Here's how the part is built. I have some questions about the finished solid (model axes, mm). A direction names the side the tool comes from. Coordinates: 2 decimals unless noted, no trailing zeros. Order: outer loops, then holes, each group sorted by start corner. A loop starts at its lowest first (then second) coordinate and runs counter-clockwise, first axis right, second up.
```python
from build123d import *

# Parameters (mm, degrees)
MODEL_R                 = 8
MODEL_R_2               = 6
MODEL_W                 = 5
MODEL_H                 = 5
SALIENTE_EXTRUIR1_DEPTH = 3


with BuildPart() as part:
    # Model → Saliente-Extruir1 (new body)
    with BuildSketch(Plane.XY):
        with BuildLine():
            Line((76.347655659, 34.880000028), (76.347655659, 24.880000028))
            Line((76.347655659, 24.880000028), (73.347655659, 24.880000028))
            Line((73.347655659, 24.880000028), (73.347655659, 6.880000028))
            Line((73.347655659, 6.880000028), (76.347655659, 6.880000028))
            Line((76.347655659, 6.880000028), (76.347655659, -3.119999972))
            Line((76.347655659, -3.119999972), (73.347655659, -3.119999972))
            Line((73.347655659, -3.119999972), (73.347655659, -14.119999972))
            Line((73.347655659, -14.119999972), (61.82755788, -14.119999972))
            Line((61.82755788, -14.119999972), (5.822580598, -14.119999972))
            ThreePointArc((5.822580598, -14.119999972), (0.393738877, -12.632215144), (-3.517289733, -8.583798005))
            ThreePointArc((-3.517289733, -8.583798005), (-0.871613495, -9.225522901), (1.80545298, -8.730822292))
            ThreePointArc((1.80545298, -8.730822292), (-2.833232138, -3.402025371), (-5.249801899, 3.236774734))
            ThreePointArc((-5.249801899, 3.236774734), (-2.74505386, 2.21277877), (-0.249855047, 3.259828604))
            ThreePointArc((-0.249855047, 3.259828604), (-3.624986156, 7.837335992), (-5.559793418, 13.185382809))
            ThreePointArc((-5.559793418, 13.185382809), (-0.86111803, 15.262797511), (2.412456901, 19.222205222))
            ThreePointArc((2.412456901, 19.222205222), (-2.310766872, 27.309140745), (-4.095322699, 36.502765137))
            ThreePointArc((-4.095322699, 36.502765137), (2.717491313, 38.336145621), (6.755388207, 44.121567597))
            ThreePointArc((6.755388207, 44.121567597), (7.57877424, 45.247904396), (8.822580598, 45.880000028))
            Line((8.822580598, 45.880000028), (11.313037594, 45.880000028))
            Line((11.313037594, 45.880000028), (73.347655659, 45.880000028))
            Line((73.347655659, 45.880000028), (73.347655659, 34.880000028))
            Line((73.347655659, 34.880000028), (76.347655659, 34.880000028))
        make_face()
        with Locations((18.822580598, 28.880000028)):
            Circle(MODEL_R, mode=Mode.SUBTRACT)
        with Locations((38.822580598, 15.880000028)):
            Circle(MODEL_R_2, mode=Mode.SUBTRACT)
        with Locations((18.822580598, 2.880000028)):
            Circle(MODEL_R, mode=Mode.SUBTRACT)
        Polygon((53.725434944, 16.464936518), (56.225434944, 20.795063537), (51.895307925, 23.295063537), (49.395307925, 18.964936518), align=None, mode=Mode.SUBTRACT)
        Polygon((49.395307925, 12.795063537), (51.895307925, 8.464936518), (56.225434944, 10.964936518), (53.725434944, 15.295063537), align=None, mode=Mode.SUBTRACT)
        with Locations((59.738574665, 23.880000028)):
            Rectangle(MODEL_W, MODEL_H, mode=Mode.SUBTRACT)
        Polygon((65.751714386, 15.295063537), (63.251714386, 10.964936518), (67.581841405, 8.464936518), (70.081841405, 12.795063537), align=None, mode=Mode.SUBTRACT)
        Polygon((70.081841405, 18.964936518), (67.581841405, 23.295063537), (63.251714386, 20.795063537), (65.751714386, 16.464936518), align=None, mode=Mode.SUBTRACT)
        with Locations((59.738574665, 7.880000028)):
            Rectangle(MODEL_W, MODEL_H, mode=Mode.SUBTRACT)
        with Locations((59.738574665, 15.880000028)):
            Rectangle(MODEL_W, MODEL_H, mode=Mode.SUBTRACT)
    extrude(amount=SALIENTE_EXTRUIR1_DEPTH)


solid = part.part
```
Q1. I need wall thicknesses on L1, parallel to X at y = 16, z = 2.45; L2, parallel to Y at x = 39, z = 2.75; L3, parallel to X at y = 23.5, z = 0.5. Which ranges of each line are inside material? Lowest first, please.
Q2. If we section it at C-C on z = 1.95: Give the number of separate pieces and of enclosed holes in the cut face, then the cut area to 3 significant figures.
Q3. If we section it at A-A on y = 28.88: Write out the boundary of the cut face in (x, z), then the cut area to 3 significant figures.
Q4. If we section it at B-B on x = 18.5: Write out the boundary of the cut face in (y, z).
Q5. We'd pull the mould along X, two halves only. Please class faces 4 (the flat face through (62.239, 24, 1)), 5 (the flat face through (45, 16, 0)), 6 (the cylindrical face through (-2.264, 27.186, 1.479)): pulls with the +X half, pulls with the -X half, needs draft (parallel to the pull), parting line crosses it, or undercut.
Q6. Will these pins go through, and if not, where does the flat tip stop? pin 1 (0.9 mm diameter, centred on x = 74.5, z = 1, fed in from +Y); pin 2 (0.9 mm diameter, centred on y = 41.5, z = 1, fed in from +X); pin 3 (1.5 mm diameter, centred on y = 3.5, z = 1, fed in from -X).
Q7. For faces 1 (the flat face through (50.663, 21.16, 1.479)), 2 (the cylindrical face through (-0.92, 15.22, 1.48)), 3 (the flat face through (75, 24.88, 1)), which set-ups out of +Z, -Z, +X, -X, +Y, -Y let a thin tool reach every point of the face, with its end or its side?
Reply:
1. L1: x = 0.02 to 32.82, 44.82 to 57.24, 62.24 to 73.35
1. L2: y = -14.12 to 9.88, 21.88 to 45.88
1. L3: x = -0.54 to 12.9, 24.74 to 57.24, 62.24 to 73.35
2. separate pieces: 1
2. enclosed holes: 10
2. area: 3,830 mm2
3. outline: (-2.85, 0) - (10.82, 0) - (10.82, 3) - (-2.85, 3) - close; (26.82, 0) - (76.35, 0) - (76.35, 3) - (26.82, 3) - close
3. area: 190 mm2
4. outline: (-14.12, 0) - (-5.11, 0) - (-5.11, 3) - (-14.12, 3) - close; (10.87, 0) - (20.89, 0) - (20.89, 3) - (10.87, 3) - close; (36.87, 0) - (45.88, 0) - (45.88, 3) - (36.87, 3) - close
5. face 4: undercut
5. face 5: needs draft
5. face 6: pulls with the -X half
6. pin 1: stops at y = 34.88
6. pin 2: stops at x = 73.35
6. pin 3: stops at x = -5.25
7. face 1: +Z, -Z
7. face 2: +Z, -Z, -X
7. face 3: +Z, -Z, +X
